from build123d import *

# Parameters (mm, degrees)
SKETCH_1_W          = 16
SKETCH_1_H          = 14
SKETCH_1_R          = 1.15
EXTRUDE_1_DEPTH     = 4
SKETCH_2_R          = 2
CUT_EXTRUDE_1_DEPTH = 2


with BuildPart() as part:
    # 스케치1 → 보스-돌출1 (new body)
    with BuildSketch(Plane(origin=(0, 0, 0), x_dir=(1, 0, 0), z_dir=(0, 1, 0))):
        Rectangle(SKETCH_1_W, SKETCH_1_H)
        with Locations((0, 4)):
            Circle(SKETCH_1_R, mode=Mode.SUBTRACT)
        with Locations((0, -4)):
            Circle(SKETCH_1_R, mode=Mode.SUBTRACT)
    extrude(amount=EXTRUDE_1_DEPTH)

    # 스케치2 → 컷-돌출1 (cut)
    with BuildSketch(Plane(origin=(0, 4, 0), x_dir=(1, 0, 0), z_dir=(0, 1, 0))):
        with Locations((0, 4)):
            Circle(SKETCH_2_R)
        with Locations((0, -4)):
            Circle(SKETCH_2_R)
    extrude(amount=-CUT_EXTRUDE_1_DEPTH, mode=Mode.SUBTRACT)


solid = part.part
Design review of the part built by this model. Coordinates are the model's own, in mm. A direction names the side the tool comes from. Give positions to 0.01 mm unless a question says otherwise; leave off trailing zeros. Write each loop counter-clockwise with the first axis right and the second up, starting at its lowest first coordinate (ties: lowest second). Pieces come first, ordered by that corner, then holes. Notation, with made-up numbers: M -39.75,63.5 L -9.75,63.5 A20 cw -9.75,96.5 Z; hole C 79.5,84.25 d4. An arc over 180 degrees is marked long. Answer as a JSON object with one key per item and string values. Group by question number.
1) Mouldability with a two-part tool opening along X and no side actions: class faces 3 (the face through (1, 2, -3)), 4 (the face through (-8, 2, 0)), 5 (the face through (-0.15, 0.99, -5.14)), 6 (the face through (0, 4, 0)) as released by +X, released by -X, zero draft, split by the parting line, or undercut.
2) Clearance check with a flat-ended pin moving along its axis: pin 1 Ø2 at (x, z) = (-0.5, 3) entering from +Y. State where the tip first meets the part, or that it passes through.
3) Tool access review of faces 1 (the face through (0, 3, -2)), 2 (the face through (0, 0, 0)): name each direction out of +Z, -Z, +X, -X, +Y, -Y from which nothing blocks a thin tool from reaching the whole face with its end or side.
4) For line 1 along Z through (x, y) = (0, 1.2); line 2 along Z through (x, y) = (0, 3.15); line 3 along X through (y, z) = (1, -4), list the stretches that pass through material, from the lowest coordinate up.
5) We need section D-D (y = 1.45). Give the boundary of the cut face in (x, z), and give its area (3 significant figures).
6) We need section B-B (z = -4). Give the boundary of the cut face in (x, y), and give its area (3 significant figures).
7) We need section A-A (x = 0). Give the boundary of the cut face in (y, z).
8) We need section C-C (y = 3.25). Give the boundary of the cut face in (x, z), and give its area (3 significant figures).
Answer key:
{
 "1": {"face 3": "undercut", "face 4": "released by -X", "face 5": "undercut", "face 6": "zero draft"},
 "2": {"pin 1": "stops at y = 4"},
 "3": {"face 1": "+Y", "face 2": "+Z, -Z, +X, -X, -Y"},
 "4": {"line 1": "z = -7 to -5.15, -2.85 to 2.85, 5.15 to 7", "line 2": "z = -7 to -6, -2 to 2, 6 to 7", "line 3": "x = -8 to -1.15, 1.15 to 8"},
 "5": {"outline": "M -8,-7 L 8,-7 L 8,7 L -8,7 Z; hole C 0,-4 d2.3; hole C 0,4 d2.3", "area": "216 mm²"},
 "6": {"outline": "M -8,0 L -1.15,0 L -1.15,2 L -2,2 L -2,4 L -8,4 Z; M 1.15,0 L 8,0 L 8,4 L 2,4 L 2,2 L 1.15,2 Z", "area": "51.4 mm²"},
 "7": {"outline": "M 0,-7 L 4,-7 L 4,-6 L 2,-6 L 2,-5.15 L 0,-5.15 Z; M 0,-2.85 L 2,-2.85 L 2,-2 L 4,-2 L 4,2 L 2,2 L 2,2.85 L 0,2.85 Z; M 0,5.15 L 2,5.15 L 2,6 L 4,6 L 4,7 L 0,7 Z"},
 "8": {"outline": "M -8,-7 L 8,-7 L 8,7 L -8,7 Z; hole C 0,-4 d4; hole C 0,4 d4", "area": "199 mm²"}
}
